Design review of the part shown in the three views and the two pictorial views. Dimensions are in mm from the part's minimum x, y and z. A direction names the side the tool comes from. Round coordinates to 2 decimals unless told otherwise and drop trailing zeros. Order: outer loops, then holes, each group sorted by start corner. A loop starts at its lowest first (then second) coordinate and runs counter-clockwise, first axis right, second up.
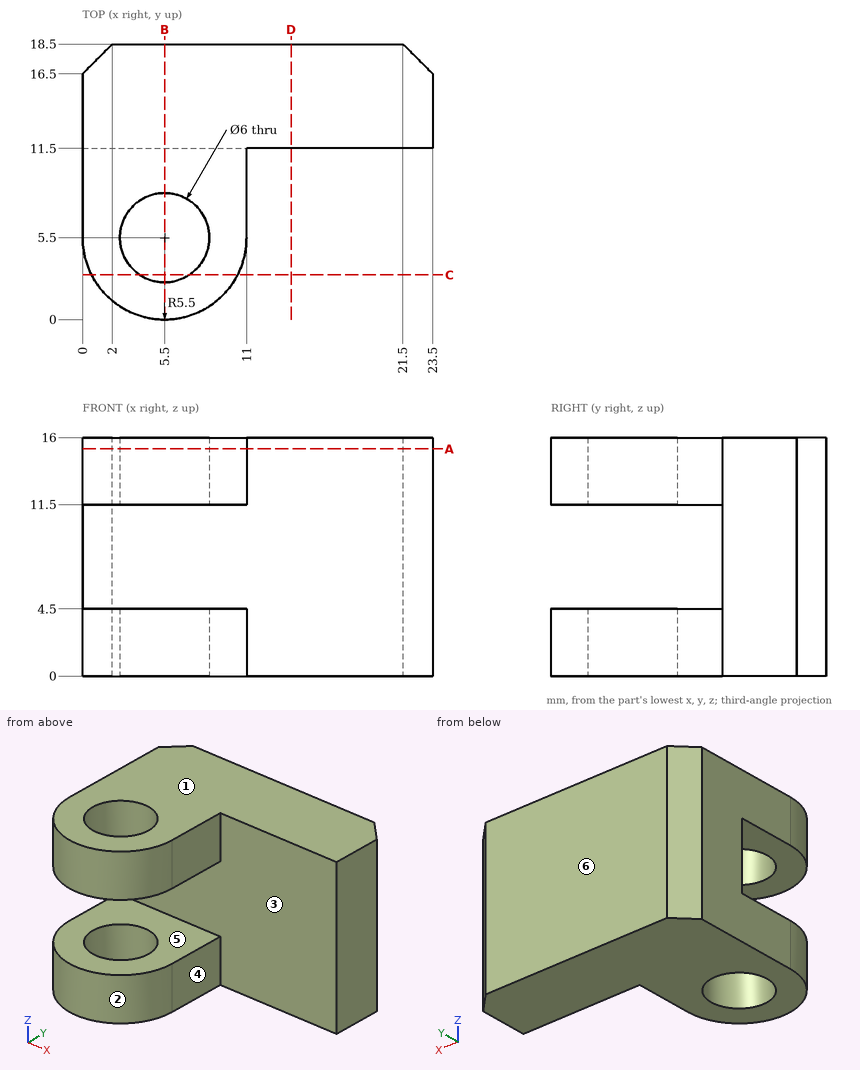
1) To check wall thickness, follow line 1 along Y through (x, z) = (5.5, 12.6); line 2 along X through (y, z) = (5.5, 1.35); line 3 along Z through (x, y) = (8, 7.5). State the ranges of each line that lie inside material, in increasing order.
Results:
line 1: y = 0 to 2.5, 8.5 to 18.5
line 2: x = 0 to 2.5, 8.5 to 11
line 3: z = 0 to 4.5, 11.5 to 16
2) Take a section at A-A on z = 15.25. Give the boundary of the cut face in (x, y), plus the area to 3 significant figures.
Results:
outline: (0, 5.5) arc R5.5 ccw to (11, 5.5) - (11, 11.5) - (23.5, 11.5) - (23.5, 16.5) - (21.5, 18.5) - (2, 18.5) - (0, 16.5) - close; hole circle Ø6 at (5.5, 5.5)
area: 246 mm2
3) The part is to be moulded in two halves that separate along Z. For the marked faces 1, 2 and 3, say which applies: released by +Z, released by -Z, zero draft, split by the parting line, or undercut.
Results:
face 1: released by +Z
face 2: zero draft
face 3: undercut
4) Take a section at C-C on y = 3. Give the boundary of the cut face in (x, z).
Results:
outline: (0.6, 0) - (3.84, 0) - (3.84, 4.5) - (0.6, 4.5) - close; (0.6, 11.5) - (3.84, 11.5) - (3.84, 16) - (0.6, 16) - close; (7.16, 0) - (10.4, 0) - (10.4, 4.5) - (7.16, 4.5) - close; (7.16, 11.5) - (10.4, 11.5) - (10.4, 16) - (7.16, 16) - close
5) Take a section at D-D on x = 14. Give the boundary of the cut face in (y, z).
Results:
outline: (11.5, 0) - (18.5, 0) - (18.5, 16) - (11.5, 16) - close
6) For the marked faces 4, 5 and 6, list the 3-axis set-ups (+Z, -Z, +X, -X, +Y, -Y) from which the entire face can be reached by the end or side of a thin tool; tool diameter is ignored.
Results:
face 4: +Z, -Z, +X, -Y
face 5: +X, -X, -Y
face 6: +Z, -Z, +X, -X, +Y
7) Take a section at B-B on x = 5.5. Give the boundary of the cut face in (y, z).
Results:
outline: (0, 0) - (2.5, 0) - (2.5, 4.5) - (0, 4.5) - close; (0, 11.5) - (2.5, 11.5) - (2.5, 16) - (0, 16) - close; (8.5, 0) - (18.5, 0) - (18.5, 16) - (8.5, 16) - (8.5, 11.5) - (11.5, 11.5) - (11.5, 4.5) - (8.5, 4.5) - close
8) Clearance check with flat-ended pins moving along their axes: P1, Ø5, axis at y = 7, z = 2, coming from the +X side; P2, Ø5.5, axis at x = 5.5, y = 5.5, coming from the +Z side; P3, Ø3, axis at x = 15, z = 12.5, coming from the -Y side. State where each tip first meets the part, or that it passes through.
Results:
P1: stops at x = 11
P2: passes through
P3: stops at y = 11.5
